Can you work these out from the model? Positions are in its coordinate system, mm. Coordinates: 2 decimals unless noted, no trailing zeros. Order: outer loops, then holes, each group sorted by start corner. A loop starts at its lowest first (then second) coordinate and runs counter-clockwise, first axis right, second up. Notation, with made-up numbers: (66, -33.75) -> (84, -33.75) arc R4 ccw to (84, -26.75) -> close; hole circle Ø3 at (54, 39). An arc over 180 degrees is marked (long way). Write item = value, one per line. Start each with the question number.
from build123d import *

# Parameters (mm, degrees)
BOSS_EXTRUDE1_DEPTH            = 11.90625
SKETCH2_W                      = 12.7
SKETCH2_H                      = 38.133687951
SKETCH2_W_2                    = 38.133687951
SKETCH2_H_2                    = 12.7
CUT_EXTRUDE1_DEPTH             = 955.226495179
F_1_4_CLEARANCE_HOLE2_D        = 6.7564
SKETCH8_W                      = 674.6875
SKETCH8_H                      = 674.6875
CUT_EXTRUDE4_DEPTH             = 955.226495179
F_5_16_0_3125_DIAMETER_HOLE1_D = 7.9375
SKETCH14_W                     = 6.35
SKETCH14_H                     = 76.233687951
SKETCH14_W_2                   = 76.233687951
SKETCH14_H_2                   = 6.35
CUT_EXTRUDE7_DEPTH             = 955.226495179


with BuildPart() as part:
    # Sketch1 → Boss-Extrude1 (new body)
    with BuildSketch(Plane(origin=(0, 0, 0), x_dir=(1, 0, 0), z_dir=(0, 1, 0))):
        with BuildLine():
            Line((-598.4875, 0), (-674.6875, 0))
            ThreePointArc((-674.6875, 0), (0, 674.6875), (674.6875, 0))
            Line((674.6875, 0), (598.4875, 0))
            ThreePointArc((598.4875, 0), (0, 598.4875), (-598.4875, 0))
        make_face()
    extrude(amount=BOSS_EXTRUDE1_DEPTH)

    # Sketch2 → Cut-Extrude1 (cut, through all)
    with BuildSketch(Plane(origin=(0, 11.90625, 0), x_dir=(1, 0, 0), z_dir=(0, 1, 0))):
        with Locations((0, 617.520656025)):
            Rectangle(SKETCH2_W, SKETCH2_H)
        with Locations((617.520656025, 0)):
            Rectangle(SKETCH2_W_2, SKETCH2_H_2)
        with Locations((0, -617.520656025)):
            Rectangle(SKETCH2_W, SKETCH2_H)
        with Locations((-617.520656025, 0)):
            Rectangle(SKETCH2_W_2, SKETCH2_H_2)
    extrude(amount=-CUT_EXTRUDE1_DEPTH, mode=Mode.SUBTRACT)

    # 1/4 Clearance Hole2 (through all)
    with Locations(Plane(origin=(0, 11.90625, 0), x_dir=(1, 0, 0), z_dir=(0, 1, 0))):
        with Locations((-31.75, 642.9375), (-31.75, 611.1875), (-611.1875, 31.75), (-642.9375, 31.75), (-567.596939292, 235.106350216), (-235.106350216, 567.596939292)):
            Hole(F_1_4_CLEARANCE_HOLE2_D / 2)

    # Sketch8 → Cut-Extrude4 (cut, through all)
    with BuildSketch(Plane(origin=(0, 11.90625, 0), x_dir=(1, 0, 0), z_dir=(0, 1, 0))):
        with Locations((337.34375, 337.34375)):
            Rectangle(SKETCH8_W, SKETCH8_H)
    extrude(amount=-CUT_EXTRUDE4_DEPTH, mode=Mode.SUBTRACT)

    # 5/16 (0.3125) Diameter Hole1 (through all)
    with Locations(Plane(origin=(0, 11.90625, 0), x_dir=(1, 0, 0), z_dir=(0, 1, 0))):
        with Locations((-247.471182654, 600.276828982), (-459.11559419, 459.11559419), (-600.276828982, 247.471182654)):
            Hole(F_5_16_0_3125_DIAMETER_HOLE1_D / 2)

    # Sketch14 → Cut-Extrude7 (cut, through all)
    with BuildSketch(Plane(origin=(0, 11.90625, 0), x_dir=(1, 0, 0), z_dir=(0, 1, 0))):
        with Locations((-3.175, 636.570656025)):
            Rectangle(SKETCH14_W, SKETCH14_H)
        with Locations((-636.570656025, 3.175)):
            Rectangle(SKETCH14_W_2, SKETCH14_H_2)
    extrude(amount=-CUT_EXTRUDE7_DEPTH, mode=Mode.SUBTRACT)


solid = part.part
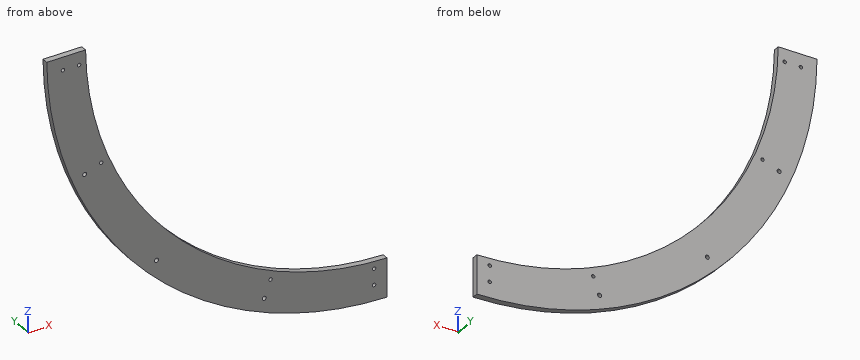
(1) If I drill on L1, parallel to Z at x = -31.75, y = 3.5; L2, parallel to Z at x = -602, y = 8.5; L3, parallel to Z at x = -610.5, y = 0.5, over which ranges is the centre line in solid material (lowest first)? Write a range as from..to.
(2) For P1, Ø1, axis at x = -270, y = 6, coming from the -Z side; P2, Ø4, axis at x = -130, y = 10.5, coming from the -Z side; P3, Ø4, axis at y = 3, z = -231.5, coming from the -X side, each with a flat end and sliding along its axis, tell me the tip position at first contact or that it passes through.
(3) Imagine slicing it at A-A (y = 2.75). Count the separate pieces of the cut face and the enclosed holes in it, plus the area to 3 significant figures.
(4) Imagine slicing it at C-C (x = -417). Write out the boundary of the cut face in (y, z), plus the area to 3 significant figures.
(5) Imagine slicing it at B-B (z = -350). Write out the boundary of the cut face in (x, y).
Result set:
q1.L1 = -673.94..-646.32, -639.56..-614.57, -607.81..-597.64
q1.L2 = -304.63..-251.05, -243.9..-6.35
q1.L3 = -287.22..-35.06, -28.44..-6.35
q2.P1 = -618.52
q2.P2 = -662.43
q2.P3 = -634.45
q3.separate_pieces = 1
q3.enclosed_holes = 9
q3.area = 74,900 mm2
q4.outline = (0, -530.39) -> (11.91, -530.39) -> (11.91, -429.3) -> (0, -429.3) -> close
q4.area = 1,200 mm2
q5.outline = (-576.8, 0) -> (-485.48, 0) -> (-485.48, 11.91) -> (-576.8, 11.91) -> close
